```python
from build123d import *

# Parameters (mm, degrees)
F0_W     = 166.958615
F0_H     = 321.350471
F1_DEPTH = 21.082
F2_T     = -2.54
F3_R     = 7.971733
F4_R     = 7.971733
F5_R     = 33.346223
F6_DEPTH = 145.542


with BuildPart() as f1:
    # F0 (on Top) → F1 (new body)
    with BuildSketch(Plane.XY):
        with Locations((-46.53474, 4.859365)):
            Rectangle(F0_W, F0_H)
    extrude(amount=F1_DEPTH)

    # F2
    f2_openings = [f1.faces().sort_by_distance(p)[0] for p in [
        (-46.534739, 4.859366, 21.082),
        (-46.534739, -155.81587, 10.541),
        (-46.534739, 165.534601, 10.541),
    ]]
    offset(amount=F2_T, openings=f2_openings)

    # F3
    f3_edges = [f1.edges().sort_by_distance(p)[0] for p in [
        (-130.014047, 165.534601, 10.541),
        (36.944568, 165.534601, 10.541),
    ]]
    fillet(f3_edges, radius=F3_R)

    # F4
    f4_edges = [f1.edges().sort_by_distance(p)[0] for p in [
        (36.944568, -155.81587, 10.541),
        (-130.014047, -155.81587, 10.541),
    ]]
    fillet(f4_edges, radius=F4_R)

    # F5 (on face) → F6 (cut)
    with BuildSketch(Plane.XY.offset(2.54)):
        with Locations((-48.913874, -52.523661)):
            Circle(F5_R)
    extrude(amount=-F6_DEPTH, mode=Mode.SUBTRACT)


solid = f1.part
```
For this review, take the finished solid that the model builds, in its own axes (mm). A direction names the side the tool comes from. Coordinates: 2 decimals unless noted, no trailing zeros. Write each loop counter-clockwise with the first axis right and the second up, starting at its lowest first coordinate (ties: lowest second). Pieces come first, ordered by that corner, then holes.
(1) Add section D-D on y = -48.5. Give the boundary of the cut face in (x, z), then the cut area to 3 significant figures.
(2) For pin 1 Ø3 at (x, y) = (15, -45) entering from +Z, flat-tipped, find the tip position at first contact; note if it passes through.
(3) Wall thickness on probe 1 along X at (y, z) = (149, 3.75); probe 2 along Z at (x, y) = (-48, 68): over which ranges is each line inside the solid? List them lowest first.
(4) Tool access review of faces 1 (the face through (36.234, 160.852, 10.689)), 2 (the face through (-48, 7, 2.54)): name each direction out of +Z, -Z, +X, -X, +Y, -Y from which nothing blocks a thin tool from reaching the whole face with its end or side.
(5) Add section A-A on z = 7.5. Give the boundary of the cut face in (x, y), then the cut area to 3 significant figures.
(6) The part is to be moulded in two halves that separate along X. For faces 3 (the face through (-127.474, 3, 12)), 4 (the face through (36.945, 3, 10)), 5 (the face through (-129.304, -151.133, 10.689)), say which applies: +X half, -X half, draft (parallel to the pull), parting line (faces both ways), or undercut.
(7) Add section C-C on x = -65.5. Give the boundary of the cut face in (y, z).
(8) Add section B-B on y = -89.5. Give the boundary of the cut face in (x, z).
Answer sheet:
1. outline: (-130.01, 0) - (-82.02, 0) - (-82.02, 2.54) - (-127.47, 2.54) - (-127.47, 21.08) - (-130.01, 21.08) - close; (-15.81, 0) - (36.94, 0) - (36.94, 21.08) - (34.4, 21.08) - (34.4, 2.54) - (-15.81, 2.54) - close
1. area: 350 mm2
2. pin 1: stops at z = 2.54
3. probe 1: x = -130.01 to -127.47, 34.4 to 36.94
3. probe 2: z = 0 to 2.54
4. face 1: +Z, -Z, +X, +Y
4. face 2: +Z, +Y, -Y
5. outline: (-130.01, -147.84) arc R7.97 ccw to (-127.47, -153.68) - (-127.47, 163.4) arc R7.97 ccw to (-130.01, 157.56) - close; (34.4, -153.68) arc R7.97 ccw to (36.94, -147.84) - (36.94, 157.56) arc R7.97 ccw to (34.4, 163.4) - close
5. area: 1,590 mm2
6. face 3: undercut
6. face 4: +X half
6. face 5: -X half
7. outline: (-155.82, 0) - (-81.45, 0) - (-81.45, 2.54) - (-155.82, 2.54) - close; (-23.59, 0) - (165.53, 0) - (165.53, 2.54) - (-23.59, 2.54) - close
8. outline: (-130.01, 0) - (36.94, 0) - (36.94, 21.08) - (34.4, 21.08) - (34.4, 2.54) - (-127.47, 2.54) - (-127.47, 21.08) - (-130.01, 21.08) - close
